Input: part model. Units: mm. Frame: model coordinates. A direction names the side the tool comes from. Give positions to 0.01 mm unless a question says otherwise; leave off trailing zeros. Order: outer loops, then holes, each group sorted by start corner. A loop starts at its lowest first (then second) coordinate and runs counter-clockwise, first axis right, second up. Notation, with made-up numbers: M 23,26.25 L 31,26.25 A22 ccw 31,57.25 Z; hole C 84.25,42 d9. An arc over 180 degrees is marked long. Use a Markdown table: item, result.
from build123d import *

# Parameters (mm, degrees)
BOSS_EXTRUDE1_DEPTH = 5.08
SKETCH3_R           = 3.175
BOSS_EXTRUDE2_DEPTH = 7.62
BOSS_EXTRUDE3_START = 2.54
SKETCH4_R           = 5.08
BOSS_EXTRUDE3_DEPTH = 2.54
SKETCH7_R           = 3.556
CUT_EXTRUDE1_DEPTH  = 5.08


with BuildPart() as part:
    # Sketch2 → Boss-Extrude1 (new body)
    with BuildSketch(Plane(origin=(0, 0, 0), x_dir=(1, 0, 0), z_dir=(0, 1, 0))):
        with BuildLine():
            Line((-50.8, -5.08), (50.8, -5.08))
            ThreePointArc((50.8, -5.08), (55.88, 0), (50.8, 5.08))
            Line((50.8, 5.08), (-50.8, 5.08))
            ThreePointArc((-50.8, 5.08), (-55.88, 0), (-50.8, -5.08))
        make_face()
    extrude(amount=BOSS_EXTRUDE1_DEPTH)

    # Sketch3 → Boss-Extrude2 (add)
    with BuildSketch(Plane.XZ):
        with Locations(Location((-50.8, 0, 0), (0, 0, 90))):
            Circle(SKETCH3_R)
        with Locations(Location((50.8, 0, 0), (0, 0, 90))):
            Circle(SKETCH3_R)
    extrude(amount=BOSS_EXTRUDE2_DEPTH)

    # Sketch4 → Boss-Extrude3 (add)
    with BuildSketch(Plane.XZ.offset(7.62).offset(BOSS_EXTRUDE3_START)):
        with Locations(Location((-50.8, 0, 0), (0, 0, 270))):
            Circle(SKETCH4_R)
        with Locations(Location((50.8, 0, 0), (0, 0, 270))):
            Circle(SKETCH4_R)
    extrude(amount=-BOSS_EXTRUDE3_DEPTH)

    # Sketch7 → Cut-Extrude1 (cut)
    with BuildSketch(Plane(origin=(0, 0, 0), x_dir=(1, 0, 0), z_dir=(0, 1, 0))):
        with Locations(Location((0, 0, 0), (0, 0, 270))):
            Circle(SKETCH7_R)
    extrude(amount=CUT_EXTRUDE1_DEPTH, mode=Mode.SUBTRACT)


solid = part.part
1) Cut plane B-B on x = 0. Return loops of the section in (y, z), and give its area (3 significant figures).
Response values:
| item | result |
|---|---|
| outline | M 0,-5.08 L 5.08,-5.08 L 5.08,-3.56 L 0,-3.56 Z; M 0,3.56 L 5.08,3.56 L 5.08,5.08 L 0,5.08 Z |
| area | 15.5 mm² |
2) Material intervals for line 1 (X direction, y = 4, z = 0); line 2 (Y direction, x = 49, z = 3.75); line 3 (Y direction, x = 29.5, z = -2), sorted ascending. Write a range as from..to.
Response values:
| item | result |
|---|---|
| line 1 | x = -55.88..-3.56, 3.56..55.88 |
| line 2 | y = -10.16..-7.62, 0..5.08 |
| line 3 | y = 0..5.08 |
3) Cut plane C-C on y = 1.5. Return loops of the section in (x, z), and give its area (3 significant figures).
Response values:
| item | result |
|---|---|
| outline | M -50.8,-5.08 L 50.8,-5.08 A5.08 ccw 50.8,5.08 L -50.8,5.08 A5.08 ccw Z; hole C 0,0 d7.11 |
| area | 1,070 mm² |
4) First-contact query: pin 1 Ø2 at (x, z) = (-6, 2) entering from -Y; pin 2 Ø2 at (y, z) = (-1.5, -0.5) entering from +X (3 decimals); pin 3 Ø1.5 at (x, y) = (43, -1) entering from -Z; pin 4 Ø4 at (y, z) = (-2.5, -1.5) entering from -X (3 decimals). Flat tips, straight axial feed; report the tip coordinate or a pass-through.
Response values:
| item | result |
|---|---|
| pin 1 | stops at y = 0 |
| pin 2 | stops at x = 53.975 |
| pin 3 | passes through |
| pin 4 | stops at x = -53.975 |
5) Reachability of faces 4 (the face through (-55.31, -8.91, -2.34)), 5 (the face through (-3.47, 2.5, -0.77)), 6 (the face through (-53.95, -3.76, -0.41)) from +Z, -Z, +X, -X, +Y, -Y: full face, straight path, thin tool, end or side. Return the list, or none.
Response values:
| item | result |
|---|---|
| face 4 | -Y |
| face 5 | +Y, -Y |
| face 6 | none |
6) Mould query, pull axis X, two halves, no side actions, for faces 1 (the face through (-1, 3, 5.08)), 2 (the face through (55.88, 2.5, 0.11)), 3 (the face through (47.65, -3.76, -0.41)). Classes: released by +X, released by -X, zero draft, split by the parting line, or undercut.
Response values:
| item | result |
|---|---|
| face 1 | zero draft |
| face 2 | released by +X |
| face 3 | undercut |
7) Cut plane D-D on y = -4.5. Return loops of the section in (x, z) (3 decimals).
Response values:
| item | result |
|---|---|
| outline | C -50.8,0 d6.35; C 50.8,0 d6.35 |
8) Cut plane A-A on z = 0. Return loops of the section in (x, y) (3 decimals).
Response values:
| item | result |
|---|---|
| outline | M -55.88,-10.16 L -45.72,-10.16 L -45.72,-7.62 L -47.625,-7.62 L -47.625,0 L -3.556,0 L -3.556,5.08 L -55.88,5.08 L -55.88,0 L -53.975,0 L -53.975,-7.62 L -55.88,-7.62 Z; M 3.556,0 L 47.625,0 L 47.625,-7.62 L 45.72,-7.62 L 45.72,-10.16 L 55.88,-10.16 L 55.88,-7.62 L 53.975,-7.62 L 53.975,0 L 55.88,0 L 55.88,5.08 L 3.556,5.08 Z |
